from build123d import *

# Parameters (mm, degrees)
BOSS_EXTRUDE1_DEPTH = 60


with BuildPart() as part:
    # Sketch1 → Boss-Extrude1 (new body)
    with BuildSketch(Plane.XY):
        with BuildLine():
            Line((0, 0), (0, -3))
            Line((0, -3), (7.034897882, -3))
            ThreePointArc((7.034897882, -3), (10.331004184, -2.441169591), (13.2587176, -0.827136649))
            ThreePointArc((13.2587176, -0.827136649), (50, 12), (86.7412824, -0.827136649))
            ThreePointArc((86.7412824, -0.827136649), (89.668995816, -2.441169591), (92.965102118, -3))
            Line((92.965102118, -3), (100, -3))
            Line((100, -3), (100, 0))
            Line((100, 0), (94, 0))
            ThreePointArc((94, 0), (90.773260722, 0.534898118), (87.891716798, 2.082369273))
            ThreePointArc((87.891716798, 2.082369273), (50, 15), (12.108283202, 2.082369273))
            ThreePointArc((12.108283202, 2.082369273), (9.226739278, 0.534898118), (6, 0))
            Line((6, 0), (0, 0))
        make_face()
    extrude(amount=BOSS_EXTRUDE1_DEPTH)


solid = part.part
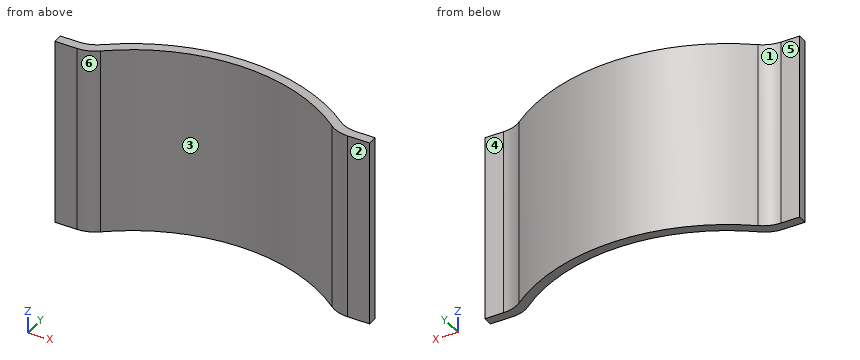
Work out the finished part from the listing and answer in its coordinate system (mm). Face numbers are marked on the shaded views. A direction names the side the tool comes from. Coordinates: 2 decimals unless noted, no trailing zeros. Loops run counter-clockwise (first coordinate to the right, second up) from the corner with the lowest first, then second, coordinate; pieces in that order, holes last. Notation, with made-up numbers: M 43.5,-21 L 61.5,-21 A20 cw 61.5,17 Z; hole C 36.5,52 d5. An arc over 180 degrees is marked long. Answer in a Markdown table with one row per item. Add a question column.
1. The mould has two halves that part along X. Classify the marked faces 1, 2 and 3: pulls with the +X half, pulls with the -X half, needs draft (parallel to the pull), parting line crosses it, or undercut.
2. Flat-ended cylindrical pins translate along their axes: P1, Ø5, axis at x = 3, z = 25.5, coming from the +Y side; P2, Ø10, axis at x = 67, z = 40.5, coming from the -Y side; P3, Ø1, axis at x = 33, z = 20, coming from the +Y side. Find the tip coordinate at first contact, or state that the pin passes through.
3. Find section C-C, the plane y = 9.75. Write down the section's boundary in (x, z).
4. Find section A-A, the plane y = -2. Write down the section's boundary in (x, z).
5. Find section B-B, the plane z = 11.5. Write down the section's boundary in (x, y).
6. A tool of negligible diameter and unlimited length cuts with its end or side. For the marked faces 4, 5 and 6, from which of +Z, -Z, +X, -X, +Y, -Y can it reach the whole face along a straight path? Write none if from no direction.
7. Consider L1, parallel to X at y = -0.5, z = 15.5; L2, parallel to X at y = 7.5, z = 12; L3, parallel to Y at x = 5, z = 52. Determine where each line is inside the solid, lowest interval first.
8. Find section D-D, the plane x = 47.5. Write down the section's boundary in (y, z).
Reported:
| question | item | result |
|---|---|---|
| 1 | face 1 | pulls with the -X half |
| 1 | face 2 | needs draft |
| 1 | face 3 | undercut |
| 2 | P1 | stops at y = 0 |
| 2 | P2 | stops at y = 7.75 |
| 2 | P3 | stops at y = 12.77 |
| 3 | outline | M 25.02,0 L 33.86,0 L 33.86,60 L 25.02,60 Z; M 66.14,0 L 74.98,0 L 74.98,60 L 66.14,60 Z |
| 4 | outline | M 0,0 L 11.39,0 L 11.39,60 L 0,60 Z; M 88.61,0 L 100,0 L 100,60 L 88.61,60 Z |
| 5 | outline | M 0,-3 L 7.03,-3 A10 ccw 13.26,-0.83 A59.03 cw 86.74,-0.83 A10 ccw 92.97,-3 L 100,-3 L 100,0 L 94,0 A10 cw 87.89,2.08 A62.03 ccw 12.11,2.08 A10 cw 6,0 L 0,0 Z |
| 6 | face 4 | +Z, -Z, +X, +Y |
| 6 | face 5 | +Z, -Z, -X, +Y |
| 6 | face 6 | +Z, -Z, -Y |
| 7 | L1 | x = 0 to 13.67, 86.33 to 100 |
| 7 | L2 | x = 20.43 to 27.39, 72.61 to 79.57 |
| 7 | L3 | y = -3 to 0 |
| 8 | outline | M 11.95,0 L 14.95,0 L 14.95,60 L 11.95,60 Z |
